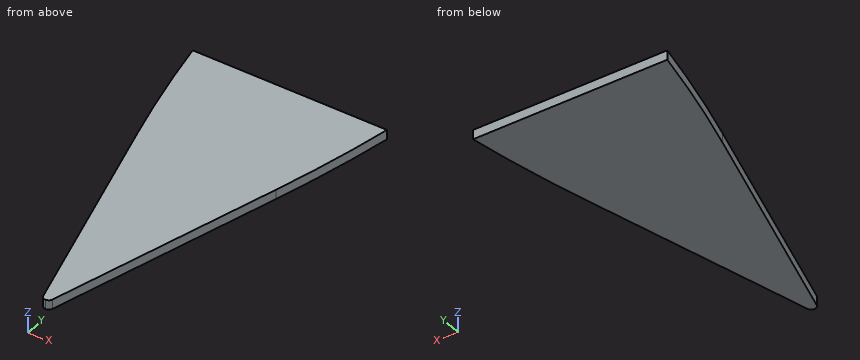
```python
from build123d import *

# Parameters (mm, degrees)
BOSS_EXTRUDE1_DEPTH = 10
SKETCH4_W           = 250.383382942
SKETCH4_H           = 630
CUT_EXTRUDE2_DEPTH  = 1008.855624389


with BuildPart() as part:
    # Sketch2 → Boss-Extrude1 (new body)
    with BuildSketch(Plane.XY):
        with BuildLine():
            Line((-75, 0), (75, 0))
            ThreePointArc((75, 0), (125.183748831, -378.01295639), (72.466338168, -755.680903745))
            Line((72.466338168, -755.680903745), (4.813443083, -996.353057902))
            ThreePointArc((4.813443083, -996.353057902), (3.01949586, -998.985303596), (0, -1000))
            ThreePointArc((0, -1000), (-3.01949586, -998.985303596), (-4.813443083, -996.353057902))
            Line((-4.813443083, -996.353057902), (-72.466338168, -755.680903745))
            ThreePointArc((-72.466338168, -755.680903745), (-125.183748831, -378.01295639), (-75, 0))
        make_face()
    extrude(amount=BOSS_EXTRUDE1_DEPTH)

    # Sketch4 → Cut-Extrude2 (cut, through all)
    with BuildSketch(Plane(origin=(0, 0, 0), x_dir=(-1, 0, 0), z_dir=(0, 0, -1))):
        with Locations((0, -315)):
            Rectangle(SKETCH4_W, SKETCH4_H)
    extrude(amount=-CUT_EXTRUDE2_DEPTH, mode=Mode.SUBTRACT)


solid = part.part
```
Verification items for the finished model (mm, model axes). Give positions to 0.01 mm unless a question says otherwise; leave off trailing zeros. Loops run counter-clockwise (first coordinate to the right, second up) from the corner with the lowest first, then second, coordinate; pieces in that order, holes last. Notation, with made-up numbers: M 67.5,-11 L 124.5,-11 A34 cw 124.5,21 Z; hole C 75,48 d10. An arc over 180 degrees is marked long. One line per question, with ' | ' between items.
Item 1: Thickness scan on line 1 (Y direction, x = -0.5, z = 6); line 2 (X direction, y = -724, z = 8); line 3 (X direction, y = -732, z = 4.25). Record the ranges inside material, lowest first. Write a range as [from, to].
Completed:
line 1: y = [-999.97, -630] | line 2: x = [-80.98, 80.98] | line 3: x = [-78.9, 78.9]
Item 2: Section check B-B, the plane y = -813. Record the cut outline in (x, z).
Completed:
outline: M -56.35,0 L 56.35,0 L 56.35,10 L -56.35,10 Z
Item 3: Section check A-A, the plane z = 6.25. Record the cut outline in (x, y).
Completed:
outline: M -101.68,-630 A1413.12 ccw -72.47,-755.68 L -4.81,-996.35 A5 ccw 4.81,-996.35 L 72.47,-755.68 A1413.12 ccw 101.68,-630 Z
Item 4: Section check C-C, the plane x = 66.5. Record the cut outline in (y, z).
Completed:
outline: M -776.91,0 L -630,0 L -630,10 L -776.91,10 Z
Item 5: Depth check by flat-ended pin: P1, Ø3, axis at x = -5.5, z = 8.5, coming from the -Y side; P2, Ø5, axis at x = -6, z = 3, coming from the -Y side; P3, Ø5, axis at y = -679.5, z = 7, coming from the -X side. Enter the tip coordinate at first touch or a pass-through.
Completed:
P1: stops at y = -998 | P2: stops at y = -998.57 | P3: stops at x = -92.17
